from build123d import *

# Parameters (mm, degrees)
F0_W      = 76.2
F0_H      = 76.2
F1_DEPTH  = 19.05
F2_R      = 25.4
F3_DEPTH  = 76.2
F4_W      = 76.2
F4_H      = 76.2
F5_DEPTH  = 19.05
F6_R      = 19.05
F7_DEPTH  = 122.174
F9_DEPTH  = 125.222
F11_DEPTH = 131.826
F13_DEPTH = 129.54
F15_DEPTH = 127


with BuildPart() as f1:
    # F0 (on Front) → F1 (new body)
    with BuildSketch(Plane.XZ):
        Rectangle(F0_W, F0_H)
    extrude(amount=F1_DEPTH)

    # F2 (on face) → F3 (join)
    with BuildSketch(Plane(origin=(0, 0, 0), x_dir=(-1, 0, 0), z_dir=(0, 1, 0))):
        Circle(F2_R)
    extrude(amount=F3_DEPTH)

    # F4 (on face) → F5 (join)
    with BuildSketch(Plane(origin=(0, 76.2, 0), x_dir=(-1, 0, 0), z_dir=(0, 1, 0))):
        Rectangle(F4_W, F4_H)
    extrude(amount=F5_DEPTH)

    # F6 (on face) → F7 (cut)
    with BuildSketch(Plane.XZ.offset(19.05)):
        Circle(F6_R)
    extrude(amount=-F7_DEPTH, mode=Mode.SUBTRACT)

    # F8 (on face) → F9 (cut)
    with BuildSketch(Plane.XZ.offset(19.05)):
        with BuildLine():
            ThreePointArc((-22.225, 28.575), (-26.14496, 34.441635), (-33.065128, 33.065128))
            Line((-33.065128, 33.065128), (-24.084872, 24.084872))
            ThreePointArc((-24.084872, 24.084872), (-22.708365, 26.14496), (-22.225, 28.575))
        make_face()
        with BuildLine():
            Line((-24.084872, 24.084872), (-33.065128, 33.065128))
            ThreePointArc((-33.065128, 33.065128), (-33.065128, 24.084872), (-24.084872, 24.084872))
        make_face()
    extrude(amount=-F9_DEPTH, mode=Mode.SUBTRACT)

    # F10 (on face) → F11 (cut)
    with BuildSketch(Plane.XZ.offset(19.05)):
        with BuildLine():
            ThreePointArc((34.925, 28.575), (34.441635, 31.00504), (33.065128, 33.065128))
            Line((33.065128, 33.065128), (24.084872, 24.084872))
            ThreePointArc((24.084872, 24.084872), (31.00504, 22.708365), (34.925, 28.575))
        make_face()
        with BuildLine():
            Line((24.084872, 24.084872), (33.065128, 33.065128))
            ThreePointArc((33.065128, 33.065128), (24.084872, 33.065128), (24.084872, 24.084872))
        make_face()
    extrude(amount=-F11_DEPTH, mode=Mode.SUBTRACT)

    # F12 (on face) → F13 (cut)
    with BuildSketch(Plane.XZ.offset(19.05)):
        with BuildLine():
            ThreePointArc((-24.084872, -24.084872), (-33.065128, -24.084872), (-33.065128, -33.065128))
            Line((-33.065128, -33.065128), (-24.084872, -24.084872))
        make_face()
        with BuildLine():
            Line((-24.084872, -24.084872), (-33.065128, -33.065128))
            ThreePointArc((-33.065128, -33.065128), (-26.14496, -34.441635), (-22.225, -28.575))
            ThreePointArc((-22.225, -28.575), (-22.708365, -26.14496), (-24.084872, -24.084872))
        make_face()
    extrude(amount=-F13_DEPTH, mode=Mode.SUBTRACT)

    # F14 (on face) → F15 (cut)
    with BuildSketch(Plane.XZ.offset(19.05)):
        with BuildLine():
            ThreePointArc((34.925, -28.575), (31.00504, -22.708365), (24.084872, -24.084872))
            Line((24.084872, -24.084872), (33.065128, -33.065128))
            ThreePointArc((33.065128, -33.065128), (34.441635, -31.00504), (34.925, -28.575))
        make_face()
        with BuildLine():
            Line((33.065128, -33.065128), (24.084872, -24.084872))
            ThreePointArc((24.084872, -24.084872), (24.084872, -33.065128), (33.065128, -33.065128))
        make_face()
    extrude(amount=-F15_DEPTH, mode=Mode.SUBTRACT)


solid = f1.part
Build history of the part. All positions in model axes, mm. A direction names the side the tool comes from. Coordinates: 2 decimals unless noted, no trailing zeros. Order: outer loops, then holes, each group sorted by start corner. A loop starts at its lowest first (then second) coordinate and runs counter-clockwise, first axis right, second up. Notation, with made-up numbers: M 27,-16 L 86,-16 A31 ccw 86,12 Z; hole C 23.25,41 d8. An arc over 180 degrees is marked long. One line per question, with ' | ' between items. Start each with the question number.
Q1. Saw through at D-D (x = -30.5). List the corners of the cut face in (y, z).
Q2. Saw through at B-B (z = 0). List the corners of the cut face in (x, y).
Q3. Two-plate mould, pull along X, no slides. Class faces 3 (the face through (-15.12, 37.3, -11.59)), 4 (the face through (-1, -9, 38.1)), 5 (the face through (38.1, 86, -1)): +X half, -X half, draft (parallel to the pull), parting line (faces both ways), or undercut.
Q4. Probe L1, parallel to X at y = 84.5, z = 28; L2, parallel to Y at x = 2, z = 32; L3, parallel to Z at x = 0, y = 51. List the from-to ranges inside material, lowest first. Write a range as from..to.
Q5. Flat gauge pins, fed straight in: pin 1 Ø4 at (y, z) = (60.5, 14.5) entering from +X; pin 2 Ø12 at (x, y) = (-22.5, 61.5) entering from +Z; pin 3 Ø1 at (x, y) = (9.5, 30) entering from -Z. Where does each tip first touch, or does it go through?
Q6. Saw through at C-C (x = 0). List the corners of the cut face in (y, z).
Q7. 3-axis set-ups, long thin cutter, end or side, ignore diameter. For faces 1 (the face through (5.506, 37.567, -24.796)), 2 (the face through (1, 86, -38.1)): which of +Z, -Z, +X, -X, +Y, -Y reach the whole face in a straight line?
Q8. Saw through at A-A (y = 84). List the corners of the cut face in (x, z) (3 decimals), then the cut area to 3 significant figures.
Check values:
1) outline: M -19.05,-38.1 L 0,-38.1 L 0,-34.63 L -19.05,-34.63 Z; M -19.05,-22.52 L 0,-22.52 L 0,22.52 L -19.05,22.52 Z; M -19.05,34.63 L 0,34.63 L 0,38.1 L -19.05,38.1 Z; M 76.2,-38.1 L 95.25,-38.1 L 95.25,-34.63 L 76.2,-34.63 Z; M 76.2,-22.52 L 95.25,-22.52 L 95.25,22.52 L 76.2,22.52 Z; M 76.2,34.63 L 95.25,34.63 L 95.25,38.1 L 76.2,38.1 Z
2) outline: M -38.1,-19.05 L -19.05,-19.05 L -19.05,95.25 L -38.1,95.25 L -38.1,76.2 L -25.4,76.2 L -25.4,0 L -38.1,0 Z; M 19.05,-19.05 L 38.1,-19.05 L 38.1,0 L 25.4,0 L 25.4,76.2 L 38.1,76.2 L 38.1,95.25 L 19.05,95.25 Z
3) face 3: undercut | face 4: draft | face 5: +X half
4) L1: x = -38.1..-34.9, -22.25..22.25, 34.9..38.1 | L2: y = -19.05..0, 76.2..95.25 | L3: z = -25.4..-19.05, 19.05..25.4
5) pin 1: stops at x = 22.11 | pin 2: stops at z = 19.31 | pin 3: stops at z = -23.75
6) outline: M -19.05,-38.1 L 0,-38.1 L 0,-25.4 L 76.2,-25.4 L 76.2,-38.1 L 95.25,-38.1 L 95.25,-19.05 L -19.05,-19.05 Z; M -19.05,19.05 L 95.25,19.05 L 95.25,38.1 L 76.2,38.1 L 76.2,25.4 L 0,25.4 L 0,38.1 L -19.05,38.1 Z
7) face 1: none | face 2: -Z, +X, -X, +Y, -Y
8) outline: M -38.1,-38.1 L 38.1,-38.1 L 38.1,38.1 L -38.1,38.1 Z; hole M -24.085,-24.085 A6.35 ccw long -22.225,-28.575 A6.35 ccw Z; hole M -24.085,24.085 A6.35 ccw -22.225,28.575 A6.35 ccw long Z; hole C 0,0 d38.1; hole M 33.065,-33.065 A6.35 ccw 34.925,-28.575 A6.35 ccw long Z; hole M 33.065,33.065 A6.35 ccw long 34.925,28.575 A6.35 ccw Z | area: 4,160 mm2
